Design review of the part built by this model. Coordinates are the model's own, in mm. A direction names the side the tool comes from. Give positions to 0.01 mm unless a question says otherwise; leave off trailing zeros. Order: outer loops, then holes, each group sorted by start corner. A loop starts at its lowest first (then second) coordinate and runs counter-clockwise, first axis right, second up. Notation, with made-up numbers: M 29,70 L 63,70 A17 ccw 63,91 Z; hole C 18,-30.5 d5. An arc over 180 degrees is marked long. Answer as a JSON object with one key per item and string values.
from build123d import *

# Parameters (mm, degrees)
SKETCH1_R           = 4
BOSS_EXTRUDE1_DEPTH = 40
SKETCH1_5_R         = 5
SKETCH1_5_R_2       = 4
BOSS_EXTRUDE2_DEPTH = 5
CUT_EXTRUDE3_DEPTH  = 1
CUT_EXTRUDE4_DEPTH  = 2


with BuildPart() as part:
    # Sketch1 → Boss-Extrude1 (new body)
    with BuildSketch(Plane.XY):
        Circle(SKETCH1_R)
    extrude(amount=BOSS_EXTRUDE1_DEPTH)

    # Sketch1<5> → Boss-Extrude2 (add)
    with BuildSketch(Plane.XY):
        Circle(SKETCH1_5_R)
        Circle(SKETCH1_5_R_2, mode=Mode.SUBTRACT)
    extrude(amount=BOSS_EXTRUDE2_DEPTH)

    # Sketch2 → Cut-Extrude3 (cut)
    with BuildSketch(Plane(origin=(0, 0, 0), x_dir=(-1, 0, 0), z_dir=(0, 0, -1))):
        Polygon((-1.600773397, 3.989869624), (-4.255715151, 0.608624385), (-2.654941754, -3.38124524), (1.600773397, -3.989869624), (4.255715151, -0.608624385), (2.654941754, 3.38124524), align=None)
    extrude(amount=-CUT_EXTRUDE3_DEPTH, mode=Mode.SUBTRACT)

    # Sketch2<2> → Cut-Extrude4 (cut)
    with BuildSketch(Plane(origin=(0, 0, 0), x_dir=(-1, 0, 0), z_dir=(0, 0, -1))):
        Polygon((-1.600773397, 3.989869624), (-4.255715151, 0.608624385), (-2.654941754, -3.38124524), (1.600773397, -3.989869624), (4.255715151, -0.608624385), (2.654941754, 3.38124524), align=None)
    extrude(amount=-CUT_EXTRUDE4_DEPTH, mode=Mode.SUBTRACT)


solid = part.part
(1) To check wall thickness, follow L1, parallel to Z at x = 3.75, y = -0.5; L2, parallel to X at y = 0.25, z = 19.5; L3, parallel to Z at x = -1.5, y = -4.5. State the ranges of each line that lie inside material, in increasing order. Write a range as from..to.
Checked values:
{"L1": "z = 2..40", "L2": "x = -3.99..3.99", "L3": "z = 0..5"}
(2) We need section A-A (y = 0). Write out the cut boundary in (x, z).
Checked values:
{"outline": "M -5,0 L -4.01,0 L -4.01,2 L 4.01,2 L 4.01,0 L 5,0 L 5,5 L 4,5 L 4,40 L -4,40 L -4,5 L -5,5 Z"}
(3) We need section C-C (z = 15). Write out the cut boundary in (x, y), plus the area to 3 significant figures.
Checked values:
{"outline": "C 0,0 d8", "area": "50.3 mm^2"}
(4) Tool access review of faces 5 (the cylindrical face through (-0.867, -3.905, 22.255)), 6 (the flat face through (0, 0, 40)), 7 (the flat face through (-3.467, 1.358, 0.986)): name each direction out of +Z, -Z, +X, -X, +Y, -Y from which nothing blocks a thin tool from reaching the whole face with its end or side.
Checked values:
{"face 5": "+Z", "face 6": "+Z, +X, -X, +Y, -Y", "face 7": "-Z"}
(5) Draft analysis for pull direction X (two halves, no side actions). For faces 1 (the flat face through (-0.56, 3.68, 0.99)), 2 (the flat face through (3.467, -1.358, 0.986)), 3 (the flat face through (0, 4, 0)), 4 (the cylindrical face through (-1.08, -4.88, 2.46)), state which applies: +X half, -X half, draft (parallel to the pull), parting line (faces both ways), or undercut.
Checked values:
{"face 1": "undercut", "face 2": "undercut", "face 3": "draft", "face 4": "parting line"}
(6) We need section B-B (x = -2). Write out the cut boundary in (y, z).
Checked values:
{"outline": "M -4.58,0 L -3.48,0 L -3.48,2 L 3.47,2 L 3.47,0 L 4.58,0 L 4.58,5 L 3.46,5 L 3.46,40 L -3.46,40 L -3.46,5 L -4.58,5 Z"}
(7) Insertion check: pin 1 (6 mm diameter, centred on y = -2, z = 27.5, fed in from -X); pin 2 (1 mm diameter, centred on x = -2.5, y = 0.5, fed in from -Z); pin 3 (6 mm diameter, centred on x = 4, z = 17, fed in from +Y). Each pin has a flat end and moves straight along its axis. Give the tip position at first contact, or say it passes through.
Checked values:
{"pin 1": "stops at x = -4", "pin 2": "stops at z = 2", "pin 3": "stops at y = 3.87"}
